Check sheet for the drawn part. Datum: minimum x, y, z corner. Units: mm. Coordinates: 2 decimals unless noted, no trailing zeros. Order: outer loops, then holes, each group sorted by start corner. A loop starts at its lowest first (then second) coordinate and runs counter-clockwise, first axis right, second up. Notation, with made-up numbers: (21.25, -33) -> (57.25, -33) arc R34 cw to (57.25, 3) -> close; hole circle Ø8 at (78.25, -7.5). An arc over 180 degrees is marked (long way). Write item = value, one per line. Start each with the question number.
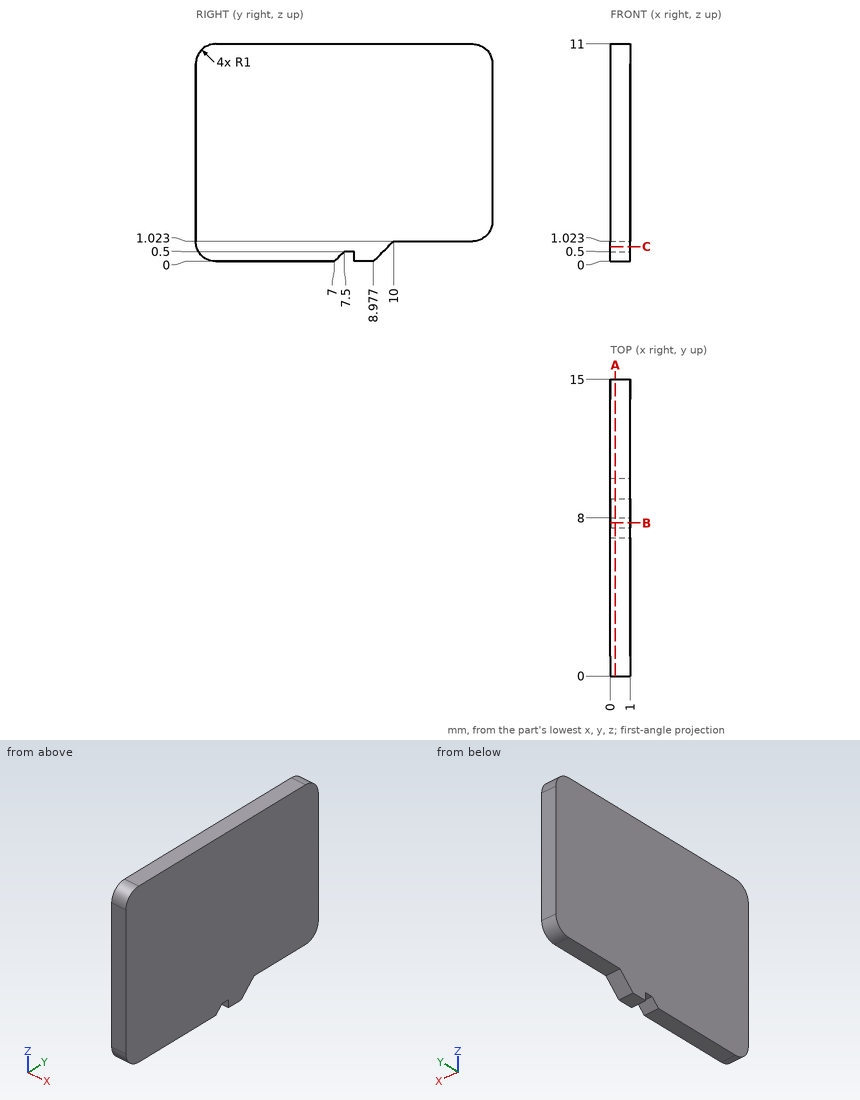
Item 1: Section check A-A (x = 0.25). Record the boundary of the cut face in (y, z), then the cut area to 3 significant figures.
Item 2: Section check C-C (z = 0.75). Record the boundary of the cut face in (x, y).
Item 3: Section check B-B (y = 7.75). Record the boundary of the cut face in (x, z).
Item 4: Thickness scan on line 1 (Z direction, x = 0.9, y = 11.75). Record the ranges inside material, lowest first.
Filled sheet:
q1.outline = (0, 1) arc R1 ccw to (1, 0) -> (7, 0) -> (7.5, 0.5) -> (8, 0.5) -> (8, 0) -> (8.98, 0) -> (10, 1.02) -> (14, 1.02) arc R1 ccw to (15, 2.02) -> (15, 10) arc R1 ccw to (14, 11) -> (1, 11) arc R1 ccw to (0, 10) -> close
q1.area = 158 mm^2
q2.outline = (0, 0.03) -> (1, 0.03) -> (1, 9.73) -> (0, 9.73) -> close
q3.outline = (0, 0.5) -> (1, 0.5) -> (1, 11) -> (0, 11) -> close
q4.line_1 = 1.02 to 11
